Can you work these out from the model? Positions are in its coordinate system, mm. Give positions to 0.01 mm unless a question says otherwise; leave off trailing zeros. Order: outer loops, then holes, each group sorted by start corner. A loop starts at its lowest first (then second) coordinate and runs counter-clockwise, first axis right, second up. Notation, with made-up numbers: (-21, 68) - (-10, 68) arc R35 cw to (-10, 103) - close; hole circle Ø5 at (-10, 62.5). An arc over 180 degrees is marked (long way). Use one line per item in the form item = value. Start each with the question number.
1) For pin 1 (1 mm diameter, centred on x = 30, y = 7.5, fed in from +Z); pin 2 (1.6 mm diameter, centred on x = 47, y = 14, fed in from +Z); pin 3 (1.6 mm diameter, centred on x = 42, y = 6.5, fed in from +Z), each with a flat end and sliding along its axis, tell me the tip position at first contact or that it passes through.
2) Please list where these lines run through material, in increasing order: probe 1 along Y at (x, z) = (5.5, 62); probe 2 along X at (y, z) = (7.7, 1.45); probe 3 along Y at (x, z) = (40.65, 0.75).
3) Suppose I cut it at C-C, the plane x = 51.5. Write out the boundary of the cut face in (y, z), and give its area (3 significant figures).
4) Suppose I cut it at B-B, the plane y = 7.7. Write out the boundary of the cut face in (x, z) (3 decimals), and give its area (3 significant figures).
5) Suppose I cut it at A-A, the plane x = 40.65. Write out the boundary of the cut face in (y, z) (3 decimals).
Autodesk Fusion 360 part; units mm, degrees
sketch "Sketch1" plane through (0, 0, 0) normal (0, 0, 1) x (1, 0, 0)
  line L0 (0, 0) -> (81.3, 0)
  line L1 (81.3, 0) -> (81.3, 15.4)
  line L2 (81.3, 15.4) -> (0, 15.4)
  line L3 (0, 15.4) -> (0, 0)
  dimension "d8" = 81.3
  dimension "d9" = 15.4
extrude "Extrude1" add sketch "Sketch1" along normal blind 5
sketch "Sketch2" plane through (0, 0, 5) normal (0, 0, 1) x (-1, 0, 0)
  line L0 (0, -15.4) -> (0, 0)
  line L1 (0, 0) -> (-81.3, 0)
  line L2 (-81.3, 0) -> (-81.3, -15.4)
  line L3 (-81.3, -15.4) -> (0, -15.4)
  circle A0 centre (-40.65, -7.7) radius 1.65
  circle A1 centre (-40.65, -7.7) radius 2.725
  dimension "d16" = 3.3
  dimension "d17" = 40.65
  dimension "d18" = 7.7
  dimension "d19" = 5.45
extrude "Extrude2" cut sketch "Sketch2" against normal blind 5 contours A0
extrude "Extrude3" cut sketch "Sketch2" against normal blind 3.1 contours A1
sketch "Sketch3" plane through (0, 0, 5) normal (0, 0, 1) x (1, 0, 0)
  line L0 (40.65, 14.9854) -> (40.65, -0.0146) construction
  line L1 (0, 15.4) -> (0, 0) construction
  line L2 (74.3, 15.4) -> (74.3, 13.4)
  line L3 (74.3, 13.4) -> (79.3, 13.4)
  line L4 (79.3, 13.4) -> (79.3, 2)
  line L5 (79.3, 2) -> (74.3, 2)
  line L6 (74.3, 2) -> (74.3, 0)
  line L7 (74.3, 0) -> (81.3, 0)
  line L8 (81.3, 0) -> (81.3, 15.4)
  line L9 (81.3, 15.4) -> (74.3, 15.4)
  line L10 (0, 0) -> (0, 15.4)
  line L11 (2, 13.4) -> (2, 2)
  line L12 (2, 2) -> (7, 2)
  line L13 (7, 13.4) -> (2, 13.4)
  line L14 (7, 0) -> (0, 0)
  line L15 (7, 15.4) -> (7, 13.4)
  line L16 (0, 15.4) -> (7, 15.4)
  line L17 (7, 2) -> (7, 0)
  line L18 (7, 15.4) -> (74.3, 15.4)
  line L19 (74.3, 15.4) -> (74.3, 13.4)
  line L20 (74.3, 13.4) -> (7, 13.4)
  line L21 (7, 13.4) -> (7, 15.4)
  line L22 (74.3, 2) -> (7, 2)
  line L23 (7, 2) -> (7, 0)
  line L24 (7, 0) -> (74.3, 0)
  line L25 (74.3, 0) -> (74.3, 2)
  point P0 (81.3, 0)
  dimension "d24" = 40.65
  dimension "d25" = 2
  dimension "d26" = 15.4
  dimension "d27" = 2
  dimension "d29" = 5
extrude "Extrude4" add sketch "Sketch3" along normal blind 95.16 contours L2 L3 L4 L5 L6 L7 L8 L9 L19 L25 | L10 L11 L12 L13 L14 L15 L16 L17 L21 L23
extrude "Extrude5" add sketch "Sketch3" along normal blind 5 contours L2 L15 L18 L19 L20 L21 | L6 L17 L22 L23 L24 L25
equation "pw = 74.8 mm"
equation "pd = 8.9 mm"
equation "ph = 158.6 mm"
equation "clearance = 1.25 mm"
equation "wall_thick = 2 mm"
equation "outer_w = 2 * clearance + 2 * wall_thick + pw"
equation "outer_d = 2 * clearance + 2 * wall_thick + pd"
equation "d8 = outer_w"
equation "d9 = outer_d"
equation "d17 = outer_w / 2"
equation "d18 = outer_d / 2"
equation "d24 = outer_w / 2"
equation "d25 = wall_thick"
equation "d26 = outer_d"
equation "d27 = wall_thick"
equation "d30 = ph * 0.6"
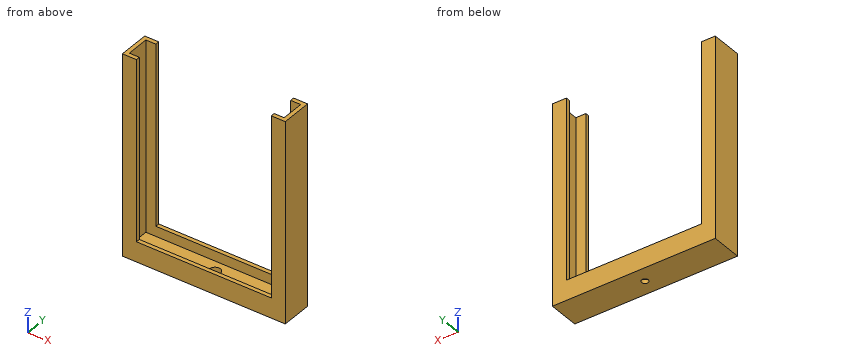
Result sheet:
q1.pin_1 = 5
q1.pin_2 = 10
q1.pin_3 = 1.9
q2.probe_1 = 0 to 2, 13.4 to 15.4
q2.probe_2 = 0 to 39, 42.3 to 81.3
q2.probe_3 = 0 to 6.05, 9.35 to 15.4
q3.outline = (0, 0) - (15.4, 0) - (15.4, 10) - (13.4, 10) - (13.4, 5) - (2, 5) - (2, 10) - (0, 10) - close
q3.area = 97.0 mm²
q4.outline = (0, 0) - (39, 0) - (39, 1.9) - (37.925, 1.9) - (37.925, 5) - (2, 5) - (2, 100.16) - (0, 100.16) - close; (42.3, 0) - (81.3, 0) - (81.3, 100.16) - (79.3, 100.16) - (79.3, 5) - (43.375, 5) - (43.375, 1.9) - (42.3, 1.9) - close
q4.area = 764 mm²
q5.outline = (0, 0) - (6.05, 0) - (6.05, 1.9) - (4.975, 1.9) - (4.975, 5) - (2, 5) - (2, 10) - (0, 10) - close; (9.35, 0) - (15.4, 0) - (15.4, 10) - (13.4, 10) - (13.4, 5) - (10.425, 5) - (10.425, 1.9) - (9.35, 1.9) - close
